Part model, mm, in its own coordinate system. A direction names the side the tool comes from. Round coordinates to 2 decimals unless told otherwise and drop trailing zeros. Loops run counter-clockwise (first coordinate to the right, second up) from the corner with the lowest first, then second, coordinate; pieces in that order, holes last.
(1) Cut at D-D on y = 0. List the corners of the cut face in (x, z), then the cut area to 4 significant figures.
(2) Probe probe 1 along X at (y, z) = (0, 2.3); probe 2 along Y at (x, z) = (0, 3.6); probe 3 along X at (y, z) = (0, 1.7). List the from-to ranges inside material, lowest first.
(3) Cut at C-C on x = -9. List the corners of the cut face in (y, z), then the cut area to 3 significant figures.
(4) Cut at B-B on y = -5.5. List the corners of the cut face in (x, z), then the cut area to 3 significant figures.
(5) Cut at A-A on x = 0. List the corners of the cut face in (y, z).
(6) Tool access for faces 4 (the face through (0, 9.758, 3)), 5 (the face through (-20.4, 1.6, 1.3)), 6 (the face through (3, -16, 2)), 7 (the face through (20.4, -1.6, 1.3)): list every direction of +Z, -Z, +X, -X, +Y, -Y with a clear straight run to the whole face (end or side of a thin tool).
(7) Flat gauge pins, fed straight in: pin 1 (3 mm diameter, centred on x = -13.5, z = 2, fed in from -Y); pin 2 (1.5 mm diameter, centred on x = 6, z = 4.5, fed in from +Y); pin 3 (1.1 mm diameter, centred on x = -20, z = 1.5, fed in from +Y). Where does each tip first touch, or does it go through?
(8) Mould opens along Y. For faces 1 (the face through (-3.45, -15.52, 3.48)), 2 (the face through (0, -21, 1)), 3 (the face through (18.3, 0, 1.3)) say: +Y half, -Y half, draft (parallel to the pull), parting line (faces both ways), or undercut.
from build123d import *

# Parameters (mm, degrees)
SKETCH_R      = 15.9
PAD_DEPTH     = 5
SKETCH001_R   = 21
SKETCH001_R_2 = 15.9
PAD001_DEPTH  = 2
POCKET_DEPTH  = 5
CHAMFER_SIZE  = 0.5


with BuildPart() as part:
    # Sketch → Pad (new body)
    with BuildSketch(Plane.XY):
        Circle(SKETCH_R)
        with BuildLine():
            Line((0.825, 8.158393), (0.825, 9.758393))
            Line((0.825, 9.758393), (-0.825, 9.758393))
            Line((-0.825, 9.758393), (-0.825, 8.158393))
            ThreePointArc((-0.825, 8.158393), (0, -8.2), (0.825, 8.158393))
        make_face(mode=Mode.SUBTRACT)
    extrude(amount=PAD_DEPTH)

    # Sketch001 → Pad001 (new body)
    with BuildSketch(Plane(origin=(0, 0, 0), x_dir=(1, 0, 0), z_dir=(0, 0, -1))):
        Circle(SKETCH001_R)
        Circle(SKETCH001_R_2, mode=Mode.SUBTRACT)
    extrude(amount=-PAD001_DEPTH)

    # Sketch002 → Pocket (cut)
    with BuildSketch(Plane.XY.offset(2)):
        with BuildLine():
            ThreePointArc((-19.9, -1.6), (-18.3, 0), (-19.9, 1.6))
            Line((-21.9, 1.6), (-19.9, 1.6))
            Line((-21.9, 1.6), (-21.9, -1.6))
            Line((-21.9, -1.6), (-19.9, -1.6))
        make_face()
        with BuildLine():
            ThreePointArc((19.9, 1.6), (18.3, 0), (19.9, -1.6))
            Line((19.9, -1.6), (21.9, -1.6))
            Line((21.9, 1.6), (21.9, -1.6))
            Line((19.9, 1.6), (21.9, 1.6))
        make_face()
    extrude(amount=-POCKET_DEPTH, mode=Mode.SUBTRACT)

    # Chamfer
    chamfer_edges = [part.edges().sort_by_distance(p)[0] for p in [
        (0.825, 8.958393, 0),
        (0, 9.758393, 0),
        (-0.825, 8.958393, 0),
        (-18.3, 0, 0),
        (18.3, 0, 0),
    ]]
    chamfer(chamfer_edges, length=CHAMFER_SIZE)


solid = part.part
Final values:
1. outline: (-18.3, 0.5) - (-17.8, 0) - (-8.2, 0) - (-8.2, 5) - (-15.9, 5) - (-15.9, 2) - (-18.3, 2) - close; (8.2, 0) - (17.8, 0) - (18.3, 0.5) - (18.3, 2) - (15.9, 2) - (15.9, 5) - (8.2, 5) - close
1. area: 86.35 mm2
2. probe 1: x = -15.9 to -8.2, 8.2 to 15.9
2. probe 2: y = -15.9 to -8.2, 9.76 to 15.9
2. probe 3: x = -18.3 to -8.2, 8.2 to 18.3
3. outline: (-18.97, 0) - (18.97, 0) - (18.97, 2) - (13.11, 2) - (13.11, 5) - (-13.11, 5) - (-13.11, 2) - (-18.97, 2) - close
3. area: 155 mm2
4. outline: (-20.27, 0) - (-6.08, 0) - (-6.08, 5) - (-14.92, 5) - (-14.92, 2) - (-20.27, 2) - close; (6.08, 0) - (20.27, 0) - (20.27, 2) - (14.92, 2) - (14.92, 5) - (6.08, 5) - close
4. area: 110 mm2
5. outline: (-21, 0) - (-8.2, 0) - (-8.2, 5) - (-15.9, 5) - (-15.9, 2) - (-21, 2) - close; (9.76, 0.5) - (10.26, 0) - (21, 0) - (21, 2) - (15.9, 2) - (15.9, 5) - (9.76, 5) - close
6. face 4: +Z, -Z
6. face 5: +Z, -Z, -X
6. face 6: +Z
6. face 7: +Z, -Z, +X
7. pin 1: stops at y = -17.23
7. pin 2: stops at y = 15.01
7. pin 3: stops at y = 7.92
8. face 1: parting line
8. face 2: -Y half
8. face 3: undercut
